Geometry: final body of the model. Coordinates: model frame, mm. A direction names the side the tool comes from. Give positions to 0.01 mm unless a question says otherwise; leave off trailing zeros. Write each loop counter-clockwise with the first axis right and the second up, starting at its lowest first coordinate (ties: lowest second). Pieces come first, ordered by that corner, then holes. Notation, with made-up numbers: (-5.75, 47) -> (39.25, 47) arc R20 cw to (39.25, 65) -> close; hole circle Ø6 at (33, -31.5). An arc over 180 degrees is marked (long way). Answer in a Markdown table with one row per item. Add a question column.
from build123d import *

# Parameters (mm, degrees)
F1_R   = 50
F1_R_2 = 49


with BuildPart() as f2:
    # F2: sweep along a path in F0
    with BuildLine(Plane.YZ) as f2_path:
        Line((0, 0), (0, -2264.158614))
        ThreePointArc((0, -2264.158614), (-19.098301, -2322.937139), (-69.098301, -2359.264266))
        Line((-69.098301, -2359.264266), (-125.371699, -2377.548601))
        ThreePointArc((-125.371699, -2377.548601), (-175.371699, -2413.875728), (-194.47, -2472.654253))
        Line((-194.47, -2472.654253), (-194.47, -2500))
    # F1 (on Top) → F2 (sweep)
    with BuildSketch(Plane.XY):
        Circle(F1_R)
        Circle(F1_R_2, mode=Mode.SUBTRACT)
    sweep(path=f2_path.line)


solid = f2.part
Q1. Access query for faces 4 (the cylindrical face through (26.34, -41.32, -1147.93)), 5 (the flat face through (33, -231, -2500)). Directions: +Z, -Z, +X, -X, +Y, -Y. A direction counts if a zero-diameter tool reaches every point of the face in a straight line with its end or side. Return the directions, or none.
Q2. Contact query for flat-ended pins moving along their axis: pin 1 Ø1.5 at (x, y) = (33.5, -127.5) entering from -Z; pin 2 Ø6 at (x, y) = (-31.5, -165) entering from +Z; pin 3 Ø5 at (x, z) = (26, -2124) entering from -Y. Output: stop coordinate, or through.
Q3. Section A-A on z = -2020. Return loops of the section in (x, y), and give its area (3 significant figures).
Q4. Line query: probe 1 along Y at (x, z) = (0, -2481); probe 2 along Y at (x, z) = (0, -874). Output: solid intervals per line, ascending. Write a range as from..to.
Q5. Pull-direction query (Y, two-part tool) for faces 1 (the flat face through (37, -33, 0)), 2 (the cylindrical face through (-10.84, -145.66, -2486.52)), 3 (the cylindrical face through (-10.622, -146.635, -2486.519)); classes: +Y half, -Y half, draft (parallel to the pull), parting line (faces both ways), or undercut.
Checks:
| question | item | result |
|---|---|---|
| 1 | face 4 | +Z |
| 1 | face 5 | -Z, +X, -X, +Y, -Y |
| 2 | pin 1 | z = -2420.06 |
| 2 | pin 2 | z = -2349.93 |
| 2 | pin 3 | y = -44.13 |
| 3 | outline | circle Ø100 at (0, 0); hole circle Ø98 at (0, 0) |
| 3 | area | 311 mm^2 |
| 4 | probe 1 | -244.47..-243.47, -145.47..-144.47 |
| 4 | probe 2 | -50..-49, 49..50 |
| 5 | face 1 | draft |
| 5 | face 2 | parting line |
| 5 | face 3 | undercut |
